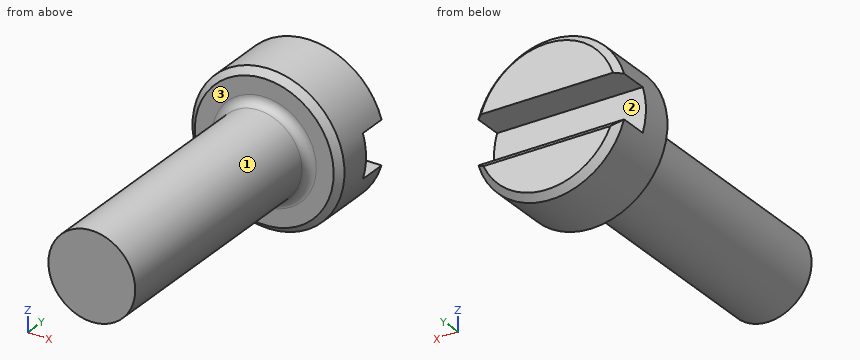
from build123d import *

# Parameters (mm, degrees)
SKETCH1_R           = 1.75
BOSS_EXTRUDE1_DEPTH = 1.7
SKETCH2_R           = 1
BOSS_EXTRUDE2_DEPTH = 6
SKETCH4_W           = 4
SKETCH4_H           = 1
CUT_EXTRUDE1_DEPTH  = 0.8
CHAMFER1_SIZE       = 0.15
FILLET1_R           = 0.2


with BuildPart() as part:
    # Sketch1 → Boss-Extrude1 (new body)
    with BuildSketch(Plane(origin=(0, 0, 0), x_dir=(1, 0, 0), z_dir=(0, 1, 0))):
        with Locations(Location((0, 0, 0), (0, 0, 270))):
            Circle(SKETCH1_R)
    extrude(amount=BOSS_EXTRUDE1_DEPTH)

    # Sketch2 → Boss-Extrude2 (add)
    with BuildSketch(Plane.XZ):
        with Locations(Location((0, 0, 0), (0, 0, 270))):
            Circle(SKETCH2_R)
    extrude(amount=BOSS_EXTRUDE2_DEPTH)

    # Sketch4 → Cut-Extrude1 (cut)
    with BuildSketch(Plane(origin=(0, 1.7, 0), x_dir=(1, 0, 0), z_dir=(0, 1, 0))):
        Rectangle(SKETCH4_W, SKETCH4_H)
    extrude(amount=-CUT_EXTRUDE1_DEPTH, mode=Mode.SUBTRACT)

    # Chamfer1
    chamfer1_edges = [part.edges().sort_by_distance(p)[0] for p in [
        (1.045825033, 1.7, 1.40312152),
        (0, 1.7, -0.5),
        (0, 0, -1.75),
        (0, 1.7, -1.75),
    ]]
    chamfer(chamfer1_edges, length=CHAMFER1_SIZE)

    # Fillet1
    fillet1_edges = [part.edges().sort_by_distance(p)[0] for p in [
        (0, 0, 1),
    ]]
    fillet(fillet1_edges, radius=FILLET1_R)


solid = part.part
Work out the finished part from the listing and answer in its coordinate system (mm). Face numbers are marked on the shaded views. Round coordinates to 2 decimals unless told otherwise and drop trailing zeros. Loops run counter-clockwise (first coordinate to the right, second up) from the corner with the lowest first, then second, coordinate; pieces in that order, holes last. Notation, with made-up numbers: (52, 59) - (87, 59) arc R10 cw to (87, 64) - close; hole circle Ø3 at (9, 31.25). An arc over 180 degrees is marked (long way). Use one line per item in the form item = value. Start each with the question number.
(1) Find section B-B on x = 0. Determine the outline of the cut face in (y, z).
(2) Consider line 1 (Y direction, x = -0.3, z = 1.2); line 2 (Z direction, x = 0.1, y = -3); line 3 (Y direction, x = 0.25, z = 0.3). Determine where each line is inside the solid, lowest interval first.
(3) Find section A-A on z = 0. Determine the outline of the cut face in (x, y).
(4) Determine the mould class of the marked faces 1, 2 and 3 for opening direction Z: +Z half, -Z half, draft (parallel to the pull), parting line (faces both ways), or undercut.
(5) Flat-ended cylindrical pins translate along their axes: P1, Ø0.5, axis at x = 0.5, y = 1, coming from the +Z side; P2, Ø0.6, axis at x = 0.5, y = 1, coming from the -Z side. Find the tip coordinate at first contact, or state that the pin passes through.
(6) Find section C-C on y = -2.25. Determine the outline of the cut face in (x, z).
(7) Find section D-D on y = 0.25. Determine the outline of the cut face in (x, z), and give its area (3 significant figures).
Answer list:
q1.outline = (-6, -1) - (-0.2, -1) arc R0.2 cw to (0, -1.2) - (0, -1.6) - (0.15, -1.75) - (1.55, -1.75) - (1.7, -1.6) - (1.7, -0.65) - (1.55, -0.5) - (0.9, -0.5) - (0.9, 0.5) - (1.7, 0.5) - (1.7, 1.6) - (1.55, 1.75) - (0.15, 1.75) - (0, 1.6) - (0, 1.2) arc R0.2 cw to (-0.2, 1) - (-6, 1) - close
q2.line_1 = 0 to 1.7
q2.line_2 = -0.99 to 0.99
q2.line_3 = -6 to 0.9
q3.outline = (-1.75, 0.15) - (-1.6, 0) - (-1.2, 0) arc R0.2 cw to (-1, -0.2) - (-1, -6) - (1, -6) - (1, -0.2) arc R0.2 cw to (1.2, 0) - (1.6, 0) - (1.75, 0.15) - (1.75, 0.9) - (-1.75, 0.9) - close
q4.face_1 = parting line
q4.face_2 = undercut
q4.face_3 = draft
q5.P1 = 1.73
q5.P2 = -1.74
q6.outline = circle Ø2 at (0, 0)
q7.outline = circle Ø3.5 at (0, 0)
q7.area = 9.62 mm^2
